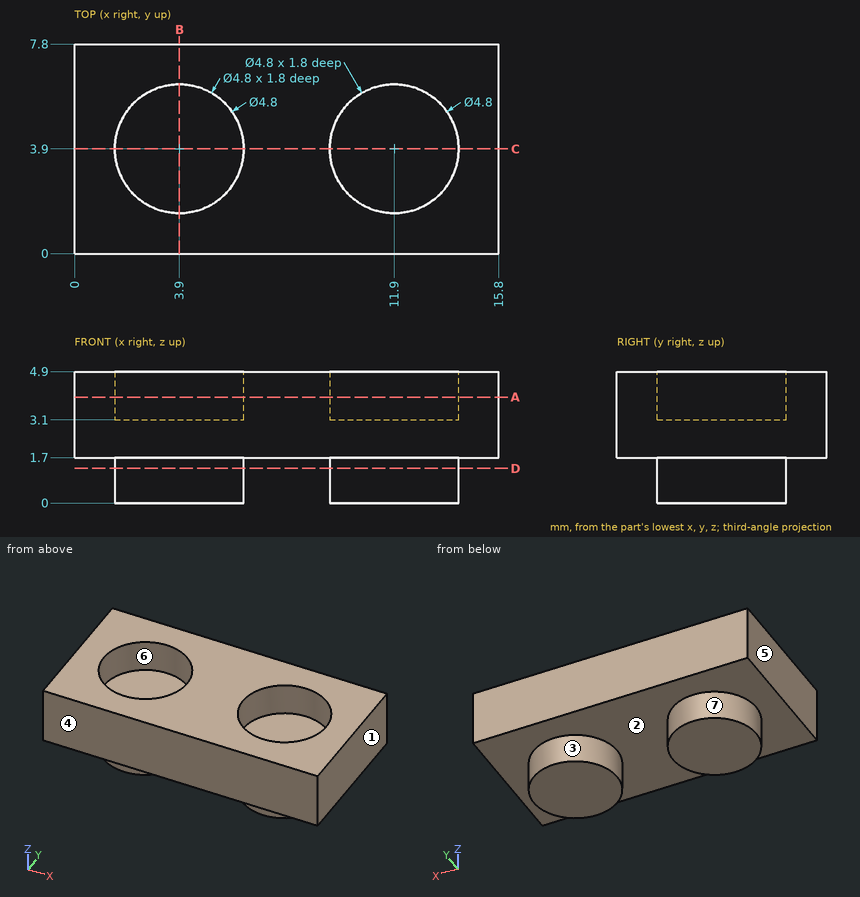
Could you check a few things on this drawing? It's one solid part, dimensions in mm from its lowest x, y, z. A direction names the side the tool comes from. Round coordinates to 2 decimals unless told otherwise and drop trailing zeros. Order: outer loops, then holes, each group sorted by start corner. A loop starts at its lowest first (then second) coordinate and runs counter-clockwise, first axis right, second up.
(1) Imagine slicing it at A-A (z = 3.95). Write out the boundary of the cut face in (x, y), plus the area to 3 significant figures.
Response values:
outline: (0, 0) - (15.8, 0) - (15.8, 7.8) - (0, 7.8) - close; hole circle Ø4.8 at (3.9, 3.9); hole circle Ø4.8 at (11.9, 3.9)
area: 87.0 mm2
(2) Which directions (+Z, -Z, +X, -X, +Y, -Y) give clear straight access to the entire face, cutting with the end or side of a thin tool? Please do the marked faces 5, 6 and 7.
Response values:
face 5: +Z, -Z, -X, +Y, -Y
face 6: +Z
face 7: -Z
(3) Please list where these lines run through material, in increasing order: line 1 along Y through (x, z) = (11.9, 4.25); line 2 along X through (y, z) = (1.75, 4.5); line 3 along X through (y, z) = (4.25, 3.8).
Response values:
line 1: y = 0 to 1.5, 6.3 to 7.8
line 2: x = 0 to 2.83, 4.97 to 10.83, 12.97 to 15.8
line 3: x = 0 to 1.53, 6.27 to 9.53, 14.27 to 15.8
(4) Imagine slicing it at B-B (x = 3.9). Write out the boundary of the cut face in (y, z).
Response values:
outline: (0, 1.7) - (1.5, 1.7) - (1.5, 0) - (6.3, 0) - (6.3, 1.7) - (7.8, 1.7) - (7.8, 4.9) - (6.3, 4.9) - (6.3, 3.1) - (1.5, 3.1) - (1.5, 4.9) - (0, 4.9) - close
(5) Imagine slicing it at D-D (z = 1.3). Write out the boundary of the cut face in (x, y).
Response values:
outline: circle Ø4.8 at (3.9, 3.9); circle Ø4.8 at (11.9, 3.9)
(6) Imagine slicing it at C-C (y = 3.9). Write out the boundary of the cut face in (x, z).
Response values:
outline: (0, 1.7) - (1.5, 1.7) - (1.5, 0) - (6.3, 0) - (6.3, 1.7) - (9.5, 1.7) - (9.5, 0) - (14.3, 0) - (14.3, 1.7) - (15.8, 1.7) - (15.8, 4.9) - (14.3, 4.9) - (14.3, 3.1) - (9.5, 3.1) - (9.5, 4.9) - (6.3, 4.9) - (6.3, 3.1) - (1.5, 3.1) - (1.5, 4.9) - (0, 4.9) - close
(7) If we mould it in two halves opening along X, with no side actions, what happens to the marked faces 1, 2, 3 and 4? For each: released by +X, released by -X, zero draft, split by the parting line, or undercut.
Response values:
face 1: released by +X
face 2: undercut
face 3: undercut
face 4: zero draft
